```python
from build123d import *

# Parameters (mm, degrees)
ESQUISSE1_W             = 157
ESQUISSE1_H             = 116
BOSS_EXTRU_1_DEPTH      = 50
ENL_V_MAT_EXTRU_1_DEPTH = 48
ESQUISSE3_R             = 18
ESQUISSE3_R_2           = 14.5
ENL_V_MAT_EXTRU_2_DEPTH = 175.679706892
ESQUISSE4_R             = 14.5
ENL_V_MAT_EXTRU_3_DEPTH = 149.722056199
ESQUISSE5_R             = 3
BOSS_EXTRU_2_DEPTH      = 5


with BuildPart() as part:
    # Esquisse1 → Boss.-Extru.1 (new body)
    with BuildSketch(Plane.XY):
        Rectangle(ESQUISSE1_W, ESQUISSE1_H)
    extrude(amount=BOSS_EXTRU_1_DEPTH)

    # Esquisse2 → Enlèv. mat.-Extru.1 (cut)
    with BuildSketch(Plane.XY):
        Polygon((-61.5, 56), (61.5, 56), (61.5, 41), (76.5, 41), (76.5, -41), (61.5, -41), (61.5, -56), (-61.5, -56), (-61.5, -41), (-76.5, -41), (-76.5, 41), (-61.5, 41), align=None)
    extrude(amount=ENL_V_MAT_EXTRU_1_DEPTH, mode=Mode.SUBTRACT)

    # Esquisse3 → Enlèv. mat.-Extru.2 (cut, through all)
    with BuildSketch(Plane(origin=(78.5, 0, 0), x_dir=(0, 0, -1), z_dir=(1, 0, 0))):
        with Locations(Location((-26, 23, 0), (0, 0, 90))):
            Circle(ESQUISSE3_R)
        with Locations(Location((-28.5, -21.5, 0), (0, 0, 90))):
            Circle(ESQUISSE3_R_2)
    extrude(amount=-ENL_V_MAT_EXTRU_2_DEPTH, mode=Mode.SUBTRACT)

    # Esquisse4 → Enlèv. mat.-Extru.3 (cut, through all)
    with BuildSketch(Plane(origin=(0, 58, 0), x_dir=(1, 0, 0), z_dir=(0, 1, 0))):
        with Locations(Location((-44, -28.5, 0), (0, 0, 270))):
            Circle(ESQUISSE4_R)
        with Locations(Location((0, -28.5, 0), (0, 0, 270))):
            Circle(ESQUISSE4_R)
        with Locations(Location((44, -28.5, 0), (0, 0, 270))):
            Circle(ESQUISSE4_R)
    extrude(amount=-ENL_V_MAT_EXTRU_3_DEPTH, mode=Mode.SUBTRACT)

    # Esquisse5 → Boss.-Extru.2 (add)
    with BuildSketch(Plane(origin=(0, 0, 48), x_dir=(-1, 0, 0), z_dir=(0, 0, -1))):
        with Locations(Location((-12.5, -21, 0), (0, 0, 180))):
            Circle(ESQUISSE5_R)
        with Locations(Location((12.5, -21, 0), (0, 0, 180))):
            Circle(ESQUISSE5_R)
        with Locations(Location((12.5, 21, 0), (0, 0, 180))):
            Circle(ESQUISSE5_R)
        with Locations(Location((-12.5, 21, 0), (0, 0, 180))):
            Circle(ESQUISSE5_R)
    extrude(amount=BOSS_EXTRU_2_DEPTH)


solid = part.part
```
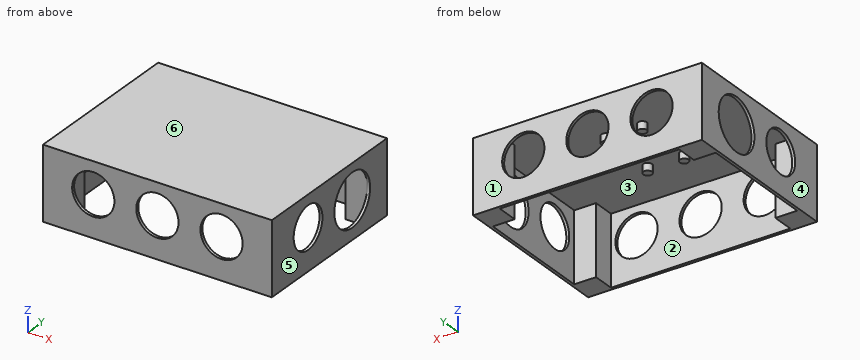
Check sheet for the modelled part. Datum: model origin and axes. Units: mm. Face numbers are marked on the shaded views. A direction names the side the tool comes from. Round coordinates to 2 decimals unless told otherwise and drop trailing zeros. Loops run counter-clockwise (first coordinate to the right, second up) from the corner with the lowest first, then second, coordinate; pieces in that order, holes last. Notation, with made-up numbers: (23.5, 77.5) - (77.5, 77.5) arc R5 ccw to (77.5, 82.5) - close; hole circle Ø6 at (35.25, 61.25). An arc over 180 degrees is marked (long way). Write item = value, one per line. Start each with the question number.
Q1. Section check D-D (x = -27). Record the boundary of the cut face in (y, z), plus the area to 3 significant figures.
Q2. Section check C-C (y = -38.5). Record the boundary of the cut face in (x, z).
Q3. Section check B-B (y = 7.5). Record the boundary of the cut face in (x, z), plus the area to 3 significant figures.
Q4. Depth check by flat-ended pin: P1, Ø6.5, axis at x = 11.5, y = -21, coming from the -Z side; P2, Ø10, axis at x = -21.5, y = -1, coming from the -Z side. Enter the tip coordinate at first touch or a pass-through.
Q5. Thickness scan on L1, parallel to X at y = -57, z = 28; L2, parallel to Z at x = 77.95, y = -21.5; L3, parallel to X at y = 37.5, z = 43.5. Record the ranges inside material, lowest first.
Q6. Release check for a two-part mould opening along X. For the marked faces 3, 4, 5 and 6 record: pulls with the +X half, pulls with the -X half, needs draft (parallel to the pull), parting line crosses it, or undercut.
Q7. Section check A-A (x = -44). Record the boundary of the cut face in (y, z), plus the area to 3 significant figures.
Q8. Access from +Z, -Z, +X, -X, +Y, -Y to the whole of each face (thin tool, end or side, straight path). Record for the marked faces 1 and 2.
Derived:
q1.outline = (-58, 0) - (-56, 0) - (-56, 48) - (56, 48) - (56, 0) - (58, 0) - (58, 50) - (-58, 50) - close
q1.area = 424 mm^2
q2.outline = (-78.5, 0) - (-76.5, 0) - (-76.5, 48) - (76.5, 48) - (76.5, 0) - (78.5, 0) - (78.5, 50) - (-78.5, 50) - close
q3.outline = (-78.5, 0) - (-76.5, 0) - (-76.5, 16.85) - (-78.5, 16.85) - close; (-78.5, 35.15) - (-76.5, 35.15) - (-76.5, 48) - (76.5, 48) - (76.5, 35.15) - (78.5, 35.15) - (78.5, 50) - (-78.5, 50) - close; (76.5, 0) - (78.5, 0) - (78.5, 16.85) - (76.5, 16.85) - close
q3.area = 433 mm^2
q4.P1 = 43
q4.P2 = 48
q5.L1 = -78.5 to -58.49, -29.51 to -14.49, 14.49 to 29.51, 58.49 to 78.5
q5.L2 = 0 to 14, 43 to 50
q5.L3 = -78.5 to -76.5, 76.5 to 78.5
q6.face_3 = undercut
q6.face_4 = pulls with the -X half
q6.face_5 = pulls with the +X half
q6.face_6 = needs draft
q7.outline = (-58, 0) - (-56, 0) - (-56, 14) - (-58, 14) - close; (-58, 43) - (-56, 43) - (-56, 48) - (56, 48) - (56, 43) - (58, 43) - (58, 50) - (-58, 50) - close; (56, 0) - (58, 0) - (58, 14) - (56, 14) - close
q7.area = 308 mm^2
q8.face_1 = +Z, -Z, +X, -X, +Y
q8.face_2 = -Z
